Autodesk Inventor part; units mm, degrees
ref_plane "YZ Plane" through (0, 0, 0) normal (1, 0, 0) x (0, 1, 0)
ref_plane "XZ Plane" through (0, 0, 0) normal (0, 1, 0) x (-1, 0, 0)
ref_plane "XY Plane" through (0, 0, 0) normal (0, 0, 1) x (1, 0, 0)
sketch "Sketch1" plane through (0, 0, 0) normal (0, 1, 0) x (-1, 0, 0)
  line L0 (15, 7.5) -> (-15, 7.5)
  line L1 (-15, 7.5) -> (-15, -7.5)
  line L2 (-15, -7.5) -> (15, -7.5)
  line L3 (15, -7.5) -> (15, 7.5)
  line L4 (15, 7.5) -> (-15, -7.5) construction
  line L5 (-15, 7.5) -> (15, -7.5) construction
  point P0 (0, 0)
  dimension "d0" = 30
  dimension "d1" = 15
extrude "Extrusion1" add sketch "Sketch1" along normal blind 5
sketch "Sketch2" plane through (0, 5, 0) normal (0, 1, 0) x (1, 0, 0)
  line L0 (5, -7.5) -> (-5, -7.5)
  line L1 (-5, -7.5) -> (-5, 7.5)
  line L2 (-5, 7.5) -> (5, 7.5)
  line L3 (5, 7.5) -> (5, -7.5)
  line L4 (5, -7.5) -> (-5, 7.5) construction
  line L5 (-5, -7.5) -> (5, 7.5) construction
  point P0 (0, 0)
  dimension "d4" = 10
  dimension "d5" = 15
extrude "Extrusion2" add sketch "Sketch2" along normal blind 30
sketch "Sketch3" plane through (-15, 0, 7.5) normal (0, 0, 1) x (1, 0, 0)
  circle A0 centre (15, 12) radius 2.1
  line L0 (0, 0) -> (30, 0)
  point P0 (15, 0)
  dimension "d8" = 4.2
  dimension "d9" = 12
extrude "Extrusion3" cut sketch "Sketch3" against normal blind 10
sketch "Sketch4" plane through (0, 5, 0) normal (0, 1, 0) x (1, 0, 0)
  circle A0 centre (-10, 2.5) radius 2.05
  line L0 (-15, 7.5) -> (-15, -7.5)
  line L1 (15, 7.5) -> (-15, 7.5)
  circle A1 centre (10, 2.5) radius 2.05
  line L2 (15, -7.5) -> (15, 7.5)
  line L3 (15, 7.5) -> (-15, 7.5)
  point P0 (0, 0)
  point P1 (-5, 7.5)
  point P2 (-10, 7.5)
  point P3 (5, 7.5)
  dimension "d12" = 4.1
  dimension "d13" = 5
  dimension "d14" = 5
  dimension "d15" = 4.1
  dimension "d16" = 5
  dimension "d17" = 5
extrude "Extrusion4" cut sketch "Sketch4" against normal through all
sketch "Sketch5" plane through (-15, 0, 7.5) normal (0, 0, 1) x (1, 0, 0)
  circle A0 centre (15, 30) radius 2.1
  line L0 (10, 35) -> (20, 35)
  point P0 (15, 0)
  dimension "d20" = 4.2
  dimension "d21" = 5
extrude "Extrusion5" cut sketch "Sketch5" against normal blind 10
sketch "Sketch8" plane through (-15, 0, 7.5) normal (0, 0, 1) x (1, 0, 0)
  circle A0 centre (15, 30) radius 2.1
  circle A1 centre (15, 12) radius 2.1
  circle A2 centre (15, 30) radius 2.1
  circle A3 centre (15, 12) radius 2.1
  circle A4 centre (15, 30) radius 2.1
  circle A5 centre (15, 12) radius 2.1
  line L0 (0, 0) -> (30, 0)
  line L1 (30, 0) -> (30, 5)
  line L2 (20, 5) -> (30, 5)
  line L3 (20, 5) -> (20, 35)
  line L4 (10, 35) -> (20, 35)
  line L5 (10, 5) -> (10, 35)
  line L6 (0, 5) -> (10, 5)
  line L7 (0, 0) -> (0, 5)
  line L8 (10, 35) -> (10, 5)
  line L9 (0, 5) -> (0, 0)
  line L10 (30, 0) -> (30, 5)
  line L11 (20, 5) -> (20, 35)
  point P0 (15, 0)
extrude "Extrusion7" cut sketch "Sketch8" against normal blind 5
sketch "Sketch9" plane through (0, 5, 0) normal (0, 1, 0) x (1, 0, 0)
  line L0 (-15, -2.5) -> (-5, -2.5)
  line L1 (-5, -2.5) -> (-5, 7.5)
  line L2 (-5, 7.5) -> (-15, 7.5)
  line L3 (-15, 7.5) -> (-15, -2.5)
  circle A0 centre (-10, 2.5) radius 2.05
  line L4 (5, -2.5) -> (15, -2.5)
  line L5 (15, -2.5) -> (15, 7.5)
  line L6 (15, 7.5) -> (5, 7.5)
  line L7 (5, 7.5) -> (5, -2.5)
  circle A1 centre (10, 2.5) radius 2.05
  point P0 (0, 0)
extrude "Extrusion8" add sketch "Sketch9" along normal blind 1
fillet "Fillet1" radius 1 20 edges at (0, 35, 2.5) (5, 35, -2.5) (0, 35, -7.5) (-5, 35, -2.5) (5, 20.5, 2.5) (5, 20.5, -7.5) (-5, 20.5, 2.5) (-5, 20.5, -7.5) (5, 6, -2.5) (-5, 6, -2.5) (-15, 6, -2.5) (-10, 6, 2.5) (10, 6, 2.5) (15, 6, -2.5) (10, 6, -7.5) (-10, 6, -7.5) (15, 3, 2.5) (15, 3, -7.5) (-15, 3, 2.5) (-15, 3, -7.5)
properties part number "al_rod_bracket" material "ABS Plastic"
CAD build for the part. Positions are in the model's coordinates, mm. A direction names the side the tool comes from. Coordinates: 2 decimals unless noted, no trailing zeros. Order: outer loops, then holes, each group sorted by start corner. A loop starts at its lowest first (then second) coordinate and runs counter-clockwise, first axis right, second up.
(1) Drill centre lines: L1, parallel to X at y = 2.55, z = -2.5; L2, parallel to Y at x = -0.5, z = -1.75; L3, parallel to X at y = 29, z = -5.75. Where is each one in solid material? Low to high.
Solution:
L1: x = -15 to -12.05, -7.95 to 7.95, 12.05 to 15
L2: y = 0 to 9.96, 14.04 to 27.96, 32.04 to 35
L3: x = -5 to 5
(2) Saw through at D-D, the plane y = 12. Write the cut outline in (x, z), and give its area (3 significant figures).
Solution:
outline: (-5, -6.5) arc R1 ccw to (-4, -7.5) - (4, -7.5) arc R1 ccw to (5, -6.5) - (5, 1.5) arc R1 ccw to (4, 2.5) - (2.1, 2.5) - (2.1, -2.5) - (-2.1, -2.5) - (-2.1, 2.5) - (-4, 2.5) arc R1 ccw to (-5, 1.5) - close
area: 78.1 mm2
(3) Which spindle directions (+Z, -Z, +X, -X, +Y, -Y) get a long thin tool onto all of the face, cutting with end or side? Do faces 1 (the face through (9.944, 5.715, -7.199)), 2 (the face through (0, 30, -2.5)), 3 (the face through (-5, 20, -2)), 4 (the face through (-4.699, 20.689, -7.215)). Say none if no direction does.
Solution:
face 1: -Z, +X, +Y
face 2: +Z
face 3: +Z, -Z, -X, +Y
face 4: -Z, -X, +Y
(4) Saw through at B-B, the plane y = 2. Write the cut outline in (x, z).
Solution:
outline: (-15, -6.5) arc R1 ccw to (-14, -7.5) - (14, -7.5) arc R1 ccw to (15, -6.5) - (15, 1.5) arc R1 ccw to (14, 2.5) - (-14, 2.5) arc R1 ccw to (-15, 1.5) - close; hole circle Ø4.1 at (-10, -2.5); hole circle Ø4.1 at (10, -2.5)
(5) Mould opens along Y. For faces 5 (the face through (14.699, 2.465, -7.215)), 6 (the face through (-0.273, 14.082, 0.035)), 7 (the face through (0.056, 34.699, -7.215)), 8 (the face through (0, 0, -2)) say: released by +Y, released by -Y, zero draft, split by the parting line, or undercut.
Solution:
face 5: zero draft
face 6: undercut
face 7: released by +Y
face 8: released by -Y
(6) Saw through at C-C, the plane z = -4. Write the cut outline in (x, y), and give its area (3 significant figures).
Solution:
outline: (-15, 0) - (-11.4, 0) - (-11.4, 6) - (-14, 6) arc R1 ccw to (-15, 5) - close; (-8.6, 0) - (8.6, 0) - (8.6, 6) - (6, 6) arc R1 cw to (5, 7) - (5, 34) arc R1 ccw to (4, 35) - (-4, 35) arc R1 ccw to (-5, 34) - (-5, 7) arc R1 cw to (-6, 6) - (-8.6, 6) - close; (11.4, 0) - (15, 0) - (15, 5) arc R1 ccw to (14, 6) - (11.4, 6) - close
area: 436 mm2
(7) Saw through at A-A, the plane x = 10. Write the cut outline in (y, z), and give its area (3 significant figures).
Solution:
outline: (0, -7.5) - (5, -7.5) arc R1 ccw to (6, -6.5) - (6, -4.55) - (0, -4.55) - close; (0, -0.45) - (6, -0.45) - (6, 1.5) arc R1 ccw to (5, 2.5) - (0, 2.5) - close
area: 35.0 mm2
(8) Pin check, flat tips, straight feed: pin 1 Ø6 at (y, z) = (17.5, 0.5) entering from -X; pin 2 Ø2.5 at (y, z) = (20.5, -4) entering from +X; pin 3 Ø2 at (x, z) = (6.5, -0.5) entering from +Y. Stop position of each tip, or through.
Solution:
pin 1: stops at x = -5
pin 2: stops at x = 5
pin 3: stops at y = 6.13
